Part model, mm, in its own coordinate system. Face numbers are marked on the shaded views. A direction names the side the tool comes from. Round coordinates to 2 decimals unless told otherwise and drop trailing zeros. Order: outer loops, then holes, each group sorted by start corner. A loop starts at its lowest first (then second) coordinate and runs counter-clockwise, first axis right, second up. Notation, with made-up numbers: (-8.75, 18.5) -> (24.25, 18.5) arc R30 ccw to (24.25, 51.5) -> close; hole circle Ø3 at (18, 17.25). An arc over 180 degrees is marked (long way). Use CSV: the item, a comma, the result in double quotes.
```python
from build123d import *

# Parameters (mm, degrees)
F1_DEPTH = 12.7


# Not quite as in the source:
# - a length typed as a fraction of an inch, garbled in the dataset ("3 / 203.2 mm" for 3/8 in), is restored


with BuildPart() as f1:
    # F0 (on Top) → F1 (new body)
    with BuildSketch(Plane.XY):
        with BuildLine():
            Line((-6, 13), (-13, 13))
            Line((-13, 13), (-13, -13))
            Line((-13, -13), (13, -13))
            Line((13, -13), (13, 13))
            Line((13, 13), (6, 13))
            Line((6, 13), (6, 4.1042417199))
            Line((6, 4.1042417199), (5.6827738736, 2.3051629565))
            ThreePointArc((5.6827738736, 2.3051629565), (5.6698549343, 2.0641245171), (5.7150699657, 1.8270126676))
            ThreePointArc((5.7150699657, 1.8270126676), (5.9283395565, 0.9245485942), (6, 0))
            ThreePointArc((6, 0), (0, -6), (-6, 0))
            ThreePointArc((-6, 0), (-5.9283395565, 0.9245485942), (-5.7150699657, 1.8270126676))
            ThreePointArc((-5.7150699657, 1.8270126676), (-5.6698549343, 2.0641245171), (-5.6827738736, 2.3051629565))
            Line((-5.6827738736, 2.3051629565), (-6, 4.1042417199))
            Line((-6, 4.1042417199), (-6, 13))
        make_face()
    extrude(amount=F1_DEPTH)


solid = f1.part
```
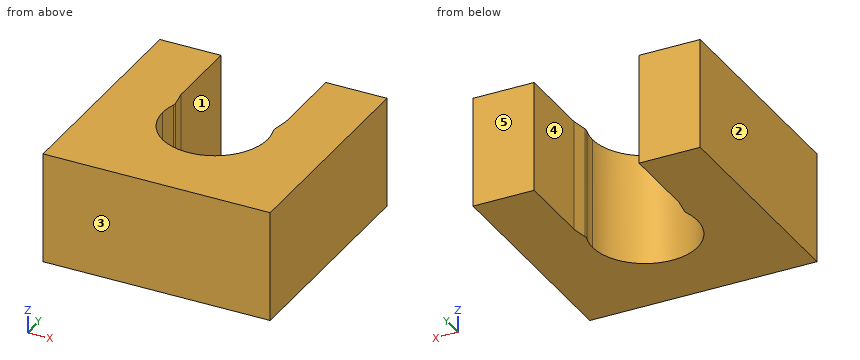
(1) Cut at D-D, the plane y = -3.25. Give the cut face in (x, z), then the cut area to 3 significant figures.
Reply:
outline,"(-13, 0) -> (-5.04, 0) -> (-5.04, 12.7) -> (-13, 12.7) -> close; (5.04, 0) -> (13, 0) -> (13, 12.7) -> (5.04, 12.7) -> close"
area,"202 mm2"
(2) Probe probe 1 along X at (y, z) = (4.25, 4.5); probe 2 along Y at (x, z) = (0, 9.5); probe 3 along X at (y, z) = (1.75, 12). List the from-to ranges inside material, lowest first. Write a range as [from, to].
Reply:
probe 1,"[-13, -6], [6, 13]"
probe 2,"[-13, -6]"
probe 3,"[-13, -5.74], [5.74, 13]"
(3) Pull direction X, two halves, no side cores. Call the marked faces 1, 2 and 3: released by +X, released by -X, zero draft, split by the parting line, or undercut.
Reply:
face 1,"undercut"
face 2,"released by -X"
face 3,"zero draft"
(4) Cut at C-C, the plane x = 0. Give the cut face in (y, z).
Reply:
outline,"(-13, 0) -> (-6, 0) -> (-6, 12.7) -> (-13, 12.7) -> close"
(5) Cut at A-A, the plane y = 4.75. Give the cut face in (x, z), then the cut area to 3 significant figures.
Reply:
outline,"(-13, 0) -> (-6, 0) -> (-6, 12.7) -> (-13, 12.7) -> close; (6, 0) -> (13, 0) -> (13, 12.7) -> (6, 12.7) -> close"
area,"178 mm2"
(6) Drop flat-ended pins along their axis: P1, Ø1.5, axis at x = 5.5, y = -7, coming from the -Z side; P2, Ø1.5, axis at x = 4.5, y = -2, coming from the +Z side. Give the stop position or say it passes through.
Reply:
P1,"z = 0"
P2,"through"
(7) Which spindle directions (+Z, -Z, +X, -X, +Y, -Y) get a long thin tool onto all of the face, cutting with end or side? Do the marked faces 4 and 5. Say none if no direction does.
Reply:
face 4,"+Z, -Z, +Y"
face 5,"+Z, -Z, +X, -X, +Y"
(8) Cut at B-B, the plane z = 4.75. Give the cut face in (x, y), then the cut area to 3 significant figures.
Reply:
outline,"(-13, -13) -> (13, -13) -> (13, 13) -> (6, 13) -> (6, 4.1) -> (5.68, 2.31) arc R1 ccw to (5.72, 1.83) arc R6 cw (long way) to (-5.72, 1.83) arc R1 ccw to (-5.68, 2.31) -> (-6, 4.1) -> (-6, 13) -> (-13, 13) -> close"
area,"465 mm2"
